Geometry: final body of the model. Coordinates: model frame, mm. A direction names the side the tool comes from. Round coordinates to 2 decimals unless told otherwise and drop trailing zeros. Write each loop counter-clockwise with the first axis right and the second up, starting at its lowest first coordinate (ties: lowest second). Pieces come first, ordered by that corner, then holes. Notation, with made-up numbers: (-34, 48.25) - (-2, 48.25) arc R37 cw to (-2, 86.25) - close; hole circle Ø6 at (81.25, 72.5). An arc over 180 degrees is marked (long way). Write each question's results on one line, items separated by ' | '.
from build123d import *

# Parameters (mm, degrees)
SKETCH2_R           = 129
SKETCH2_R_2         = 17.5
SKETCH2_R_3         = 5
BOSS_EXTRUDE1_DEPTH = 47.5
SKETCH3_W           = 75
SKETCH3_H           = 108.188611699


with BuildPart() as part:
    # Sketch2 → Boss-Extrude1 (new, symmetric)
    # profile 1 of 6: a face of its own
    with BuildSketch(Plane.YZ):
        with Locations(Location((0, 0, 0), (0, 0, 270))):
            Circle(SKETCH2_R)
        with BuildLine():
            Line((-7.5, 124.774797135), (-7.5, 15.811388301))
            ThreePointArc((-7.5, 15.811388301), (0, 17.5), (7.5, 15.811388301))
            Line((7.5, 15.811388301), (7.5, 124.774797135))
            ThreePointArc((7.5, 124.774797135), (73.473156537, 101.127124297), (116.350256427, 45.690456657))
            Line((116.350256427, 45.690456657), (12.719896417, 12.018911562))
            ThreePointArc((12.719896417, 12.018911562), (16.261122152, 6.467295134), (17.5, 0))
            ThreePointArc((17.5, 0), (17.463750289, -1.125800087), (17.355151333, -2.246936183))
            Line((17.355151333, -2.246936183), (120.985511342, 31.424608912))
            ThreePointArc((120.985511342, 31.424608912), (118.882064537, -38.627124297), (79.408413071, -96.536541959))
            Line((79.408413071, -96.536541959), (15.361328319, -8.383292448))
            ThreePointArc((15.361328319, -8.383292448), (10.286241915, -14.157797402), (3.226073404, -17.200071232))
            Line((3.226073404, -17.200071232), (67.273158156, -105.353320744))
            ThreePointArc((67.273158156, -105.353320744), (0, -125), (-67.273158156, -105.353320744))
            Line((-67.273158156, -105.353320744), (-3.226073404, -17.200071232))
            ThreePointArc((-3.226073404, -17.200071232), (-10.286241915, -14.157797402), (-15.361328319, -8.383292448))
            Line((-15.361328319, -8.383292448), (-79.408413071, -96.536541959))
            ThreePointArc((-79.408413071, -96.536541959), (-118.882064537, -38.627124297), (-120.985511342, 31.424608912))
            Line((-120.985511342, 31.424608912), (-17.355151333, -2.246936183))
            ThreePointArc((-17.355151333, -2.246936183), (-16.643489035, 5.407797402), (-12.719896417, 12.018911562))
            Line((-12.719896417, 12.018911562), (-116.350256427, 45.690456657))
            ThreePointArc((-116.350256427, 45.690456657), (-73.473156537, 101.127124297), (-7.5, 124.774797135))
        make_face(mode=Mode.SUBTRACT)
    # profile 2 of 6: a face of its own
    with BuildSketch(Plane.YZ):
        with Locations(Location((0, 0, 0), (0, 0, 270))):
            Circle(SKETCH2_R)
        with BuildLine():
            Line((-7.5, 124.774797135), (-7.5, 15.811388301))
            ThreePointArc((-7.5, 15.811388301), (0, 17.5), (7.5, 15.811388301))
            Line((7.5, 15.811388301), (7.5, 124.774797135))
            ThreePointArc((7.5, 124.774797135), (73.473156537, 101.127124297), (116.350256427, 45.690456657))
            Line((116.350256427, 45.690456657), (12.719896417, 12.018911562))
            ThreePointArc((12.719896417, 12.018911562), (16.261122152, 6.467295134), (17.5, 0))
            ThreePointArc((17.5, 0), (17.463750289, -1.125800087), (17.355151333, -2.246936183))
            Line((17.355151333, -2.246936183), (120.985511342, 31.424608912))
            ThreePointArc((120.985511342, 31.424608912), (118.882064537, -38.627124297), (79.408413071, -96.536541959))
            Line((79.408413071, -96.536541959), (15.361328319, -8.383292448))
            ThreePointArc((15.361328319, -8.383292448), (10.286241915, -14.157797402), (3.226073404, -17.200071232))
            Line((3.226073404, -17.200071232), (67.273158156, -105.353320744))
            ThreePointArc((67.273158156, -105.353320744), (0, -125), (-67.273158156, -105.353320744))
            Line((-67.273158156, -105.353320744), (-3.226073404, -17.200071232))
            ThreePointArc((-3.226073404, -17.200071232), (-10.286241915, -14.157797402), (-15.361328319, -8.383292448))
            Line((-15.361328319, -8.383292448), (-79.408413071, -96.536541959))
            ThreePointArc((-79.408413071, -96.536541959), (-118.882064537, -38.627124297), (-120.985511342, 31.424608912))
            Line((-120.985511342, 31.424608912), (-17.355151333, -2.246936183))
            ThreePointArc((-17.355151333, -2.246936183), (-16.643489035, 5.407797402), (-12.719896417, 12.018911562))
            Line((-12.719896417, 12.018911562), (-116.350256427, 45.690456657))
            ThreePointArc((-116.350256427, 45.690456657), (-73.473156537, 101.127124297), (-7.5, 124.774797135))
        make_face(mode=Mode.SUBTRACT)
    # profile 3 of 6: a face of its own
    with BuildSketch(Plane.YZ):
        with Locations(Location((0, 0, 0), (0, 0, 270))):
            Circle(SKETCH2_R)
        with BuildLine():
            Line((-7.5, 124.774797135), (-7.5, 15.811388301))
            ThreePointArc((-7.5, 15.811388301), (0, 17.5), (7.5, 15.811388301))
            Line((7.5, 15.811388301), (7.5, 124.774797135))
            ThreePointArc((7.5, 124.774797135), (73.473156537, 101.127124297), (116.350256427, 45.690456657))
            Line((116.350256427, 45.690456657), (12.719896417, 12.018911562))
            ThreePointArc((12.719896417, 12.018911562), (16.261122152, 6.467295134), (17.5, 0))
            ThreePointArc((17.5, 0), (17.463750289, -1.125800087), (17.355151333, -2.246936183))
            Line((17.355151333, -2.246936183), (120.985511342, 31.424608912))
            ThreePointArc((120.985511342, 31.424608912), (118.882064537, -38.627124297), (79.408413071, -96.536541959))
            Line((79.408413071, -96.536541959), (15.361328319, -8.383292448))
            ThreePointArc((15.361328319, -8.383292448), (10.286241915, -14.157797402), (3.226073404, -17.200071232))
            Line((3.226073404, -17.200071232), (67.273158156, -105.353320744))
            ThreePointArc((67.273158156, -105.353320744), (0, -125), (-67.273158156, -105.353320744))
            Line((-67.273158156, -105.353320744), (-3.226073404, -17.200071232))
            ThreePointArc((-3.226073404, -17.200071232), (-10.286241915, -14.157797402), (-15.361328319, -8.383292448))
            Line((-15.361328319, -8.383292448), (-79.408413071, -96.536541959))
            ThreePointArc((-79.408413071, -96.536541959), (-118.882064537, -38.627124297), (-120.985511342, 31.424608912))
            Line((-120.985511342, 31.424608912), (-17.355151333, -2.246936183))
            ThreePointArc((-17.355151333, -2.246936183), (-16.643489035, 5.407797402), (-12.719896417, 12.018911562))
            Line((-12.719896417, 12.018911562), (-116.350256427, 45.690456657))
            ThreePointArc((-116.350256427, 45.690456657), (-73.473156537, 101.127124297), (-7.5, 124.774797135))
        make_face(mode=Mode.SUBTRACT)
    # profile 4 of 6: a face of its own
    with BuildSketch(Plane.YZ):
        with Locations(Location((0, 0, 0), (0, 0, 270))):
            Circle(SKETCH2_R)
        with BuildLine():
            Line((-7.5, 124.774797135), (-7.5, 15.811388301))
            ThreePointArc((-7.5, 15.811388301), (0, 17.5), (7.5, 15.811388301))
            Line((7.5, 15.811388301), (7.5, 124.774797135))
            ThreePointArc((7.5, 124.774797135), (73.473156537, 101.127124297), (116.350256427, 45.690456657))
            Line((116.350256427, 45.690456657), (12.719896417, 12.018911562))
            ThreePointArc((12.719896417, 12.018911562), (16.261122152, 6.467295134), (17.5, 0))
            ThreePointArc((17.5, 0), (17.463750289, -1.125800087), (17.355151333, -2.246936183))
            Line((17.355151333, -2.246936183), (120.985511342, 31.424608912))
            ThreePointArc((120.985511342, 31.424608912), (118.882064537, -38.627124297), (79.408413071, -96.536541959))
            Line((79.408413071, -96.536541959), (15.361328319, -8.383292448))
            ThreePointArc((15.361328319, -8.383292448), (10.286241915, -14.157797402), (3.226073404, -17.200071232))
            Line((3.226073404, -17.200071232), (67.273158156, -105.353320744))
            ThreePointArc((67.273158156, -105.353320744), (0, -125), (-67.273158156, -105.353320744))
            Line((-67.273158156, -105.353320744), (-3.226073404, -17.200071232))
            ThreePointArc((-3.226073404, -17.200071232), (-10.286241915, -14.157797402), (-15.361328319, -8.383292448))
            Line((-15.361328319, -8.383292448), (-79.408413071, -96.536541959))
            ThreePointArc((-79.408413071, -96.536541959), (-118.882064537, -38.627124297), (-120.985511342, 31.424608912))
            Line((-120.985511342, 31.424608912), (-17.355151333, -2.246936183))
            ThreePointArc((-17.355151333, -2.246936183), (-16.643489035, 5.407797402), (-12.719896417, 12.018911562))
            Line((-12.719896417, 12.018911562), (-116.350256427, 45.690456657))
            ThreePointArc((-116.350256427, 45.690456657), (-73.473156537, 101.127124297), (-7.5, 124.774797135))
        make_face(mode=Mode.SUBTRACT)
    # profile 5 of 6: a face of its own
    with BuildSketch(Plane.YZ):
        with Locations(Location((0, 0, 0), (0, 0, 270))):
            Circle(SKETCH2_R)
        with BuildLine():
            Line((-7.5, 124.774797135), (-7.5, 15.811388301))
            ThreePointArc((-7.5, 15.811388301), (0, 17.5), (7.5, 15.811388301))
            Line((7.5, 15.811388301), (7.5, 124.774797135))
            ThreePointArc((7.5, 124.774797135), (73.473156537, 101.127124297), (116.350256427, 45.690456657))
            Line((116.350256427, 45.690456657), (12.719896417, 12.018911562))
            ThreePointArc((12.719896417, 12.018911562), (16.261122152, 6.467295134), (17.5, 0))
            ThreePointArc((17.5, 0), (17.463750289, -1.125800087), (17.355151333, -2.246936183))
            Line((17.355151333, -2.246936183), (120.985511342, 31.424608912))
            ThreePointArc((120.985511342, 31.424608912), (118.882064537, -38.627124297), (79.408413071, -96.536541959))
            Line((79.408413071, -96.536541959), (15.361328319, -8.383292448))
            ThreePointArc((15.361328319, -8.383292448), (10.286241915, -14.157797402), (3.226073404, -17.200071232))
            Line((3.226073404, -17.200071232), (67.273158156, -105.353320744))
            ThreePointArc((67.273158156, -105.353320744), (0, -125), (-67.273158156, -105.353320744))
            Line((-67.273158156, -105.353320744), (-3.226073404, -17.200071232))
            ThreePointArc((-3.226073404, -17.200071232), (-10.286241915, -14.157797402), (-15.361328319, -8.383292448))
            Line((-15.361328319, -8.383292448), (-79.408413071, -96.536541959))
            ThreePointArc((-79.408413071, -96.536541959), (-118.882064537, -38.627124297), (-120.985511342, 31.424608912))
            Line((-120.985511342, 31.424608912), (-17.355151333, -2.246936183))
            ThreePointArc((-17.355151333, -2.246936183), (-16.643489035, 5.407797402), (-12.719896417, 12.018911562))
            Line((-12.719896417, 12.018911562), (-116.350256427, 45.690456657))
            ThreePointArc((-116.350256427, 45.690456657), (-73.473156537, 101.127124297), (-7.5, 124.774797135))
        make_face(mode=Mode.SUBTRACT)
    # profile 6 of 6: a face of its own
    with BuildSketch(Plane.YZ):
        Circle(SKETCH2_R_2)
        with Locations(Location((0, 0, 0), (0, 0, 270))):
            Circle(SKETCH2_R_3, mode=Mode.SUBTRACT)
    extrude(amount=BOSS_EXTRUDE1_DEPTH, both=True)

    # Sketch3 → Cut-Revolve1 (revolve, cut)
    with BuildSketch(Plane(origin=(0, 0, 0), x_dir=(-1, 0, 0), z_dir=(0, 1, 0)), mode=Mode.PRIVATE) as cut_revolve1_sk:
        with Locations((0, 69.905694151)):
            Rectangle(SKETCH3_W, SKETCH3_H)
    revolve(cut_revolve1_sk.sketch.rotate(Axis((1000, 0, 0), (-1, 0, 0)), 180), axis=Axis((1000, 0, 0), (-1, 0, 0)), mode=Mode.SUBTRACT)


solid = part.part
Q1. Section query C-C, the plane z = -112.5. Return loops of the section in (x, y).
Answer block:
outline: (-47.5, -63.12) - (47.5, -63.12) - (47.5, -54.49) - (-47.5, -54.49) - close; (-47.5, 54.49) - (47.5, 54.49) - (47.5, 63.12) - (-47.5, 63.12) - close
Q2. Section query B-B, the plane y = 0. Return loops of the section in (x, z).
Answer block:
outline: (-47.5, -129) - (47.5, -129) - (47.5, -125) - (-47.5, -125) - close; (-47.5, -17.5) - (-37.5, -17.5) - (-37.5, -15.81) - (37.5, -15.81) - (37.5, -17.5) - (47.5, -17.5) - (47.5, -5) - (-47.5, -5) - close; (-47.5, 5) - (47.5, 5) - (47.5, 129) - (-47.5, 129) - close; hole (-37.5, 15.81) - (37.5, 15.81) - (37.5, 124) - (-37.5, 124) - close
Q3. Pin query (flat end, axial travel): pin 1 (1 mm diameter, centred on x = 29, y = 100.5, fed in from +Z); pin 2 (2 mm diameter, centred on x = 6, z = 39, fed in from +Y); pin 3 (1.5 mm diameter, centred on x = 3, y = 88, fed in from -Z). Return the tip coordinate at first contact, or that it passes through.
Answer block:
pin 1: z = 81.49 | pin 2: y = 123.28 | pin 3: z = -95.02
Q4. Ray query, line 1 along Y through (x, z) = (5, 0); line 2 along X through (y, z) = (67.5, -80.5); line 3 along Z through (x, y) = (-29.5, -9). Return the intervals inside material, ascending.
Answer block:
line 1: -129 to -125, -15.81 to -5, 5 to 15.81, 125 to 129 | line 2: -47.5 to -37.5, 37.5 to 47.5 | line 3: -128.69 to -124.68, -13 to 13, 124.68 to 128.69
Q5. Section query A-A, the plane x = -21. Return loops of the section in (y, z), plus the area to 3 significant figures.
Answer block:
outline: circle Ø258 at (0, 0); circle Ø31.62 at (0, 0); hole (-120.99, 31.42) arc R125 ccw to (-79.41, -96.54) - (-78.82, -95.73) arc R124 ccw to (-66.68, -104.54) - (-67.27, -105.35) arc R125 ccw to (67.27, -105.35) - (66.68, -104.54) arc R124 ccw to (78.82, -95.73) - (79.41, -96.54) arc R125 ccw to (120.99, 31.42) - (120.03, 31.12) arc R124 ccw to (115.4, 45.38) - (116.35, 45.69) arc R125 ccw to (7.5, 124.77) - (7.5, 123.77) arc R124 ccw to (-7.5, 123.77) - (-7.5, 124.77) arc R125 ccw to (-116.35, 45.69) - (-115.4, 45.38) arc R124 ccw to (-120.03, 31.12) - close; hole circle Ø10 at (0, 0) | area: 3,970 mm2
Q6. Mould query, pull axis X, two halves, no side actions, for faces 3 (the cylindrical face through (-0.525, 117.898, 38.418)), 4 (the cylindrical face through (0.665, 38.748, -123.043)), 5 (the flat face through (-47.5, -10, 10)). Classes: pulls with the +X half, pulls with the -X half, needs draft (parallel to the pull), parting line crosses it, or undercut.
Answer block:
face 3: undercut | face 4: needs draft | face 5: pulls with the -X half
Q7. Section query D-D, the plane y = -50. Return loops of the section in (x, z).
Answer block:
outline: (-47.5, -118.92) - (47.5, -118.92) - (47.5, -114.56) - (-47.5, -114.56) - close; (-47.5, -81.58) - (-37.5, -81.58) - (-37.5, -56.06) - (-47.5, -56.06) - close; (-47.5, 8.36) - (-37.5, 8.36) - (-37.5, 24.13) - (-47.5, 24.13) - close; (-47.5, 114.56) - (47.5, 114.56) - (47.5, 118.92) - (-47.5, 118.92) - close; (37.5, -81.58) - (47.5, -81.58) - (47.5, -56.06) - (37.5, -56.06) - close; (37.5, 8.36) - (47.5, 8.36) - (47.5, 24.13) - (37.5, 24.13) - close
Q8. Access query for faces 1 (the cylindrical face through (-0.52, -72.8, -100.38)), 2 (the cylindrical face through (-42.4, 0, -17.5)). Directions: +Z, -Z, +X, -X, +Y, -Y. A direction counts if a zero-diameter tool reaches every point of the face in a straight line with its end or side. Return the directions, or none.
Answer block:
face 1: none | face 2: +X, -X
